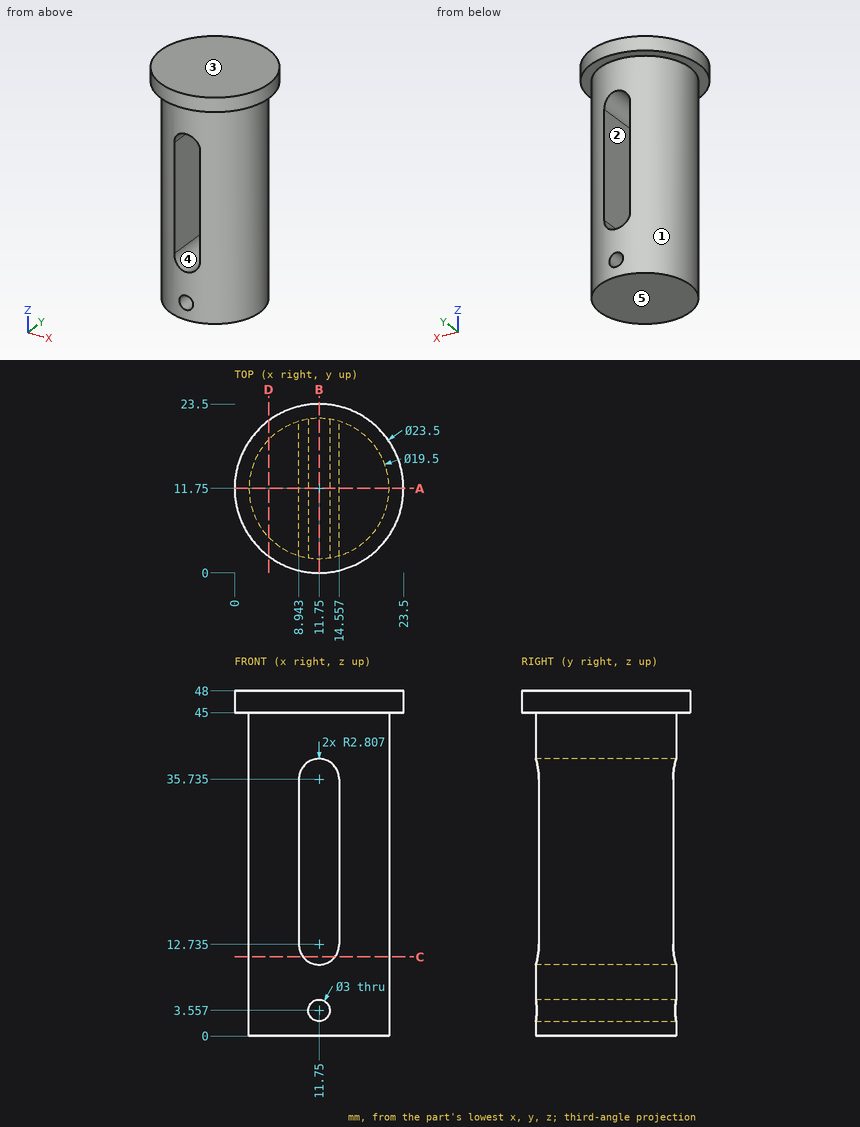
Part print with two shaded views. Sizes in mm from the minimum x, y, z corner. A direction names the side the tool comes from. Coordinates: 2 decimals unless noted, no trailing zeros. Write each loop counter-clockwise with the first axis right and the second up, starting at its lowest first coordinate (ties: lowest second). Pieces come first, ordered by that corner, then holes. Notation, with made-up numbers: (86, 30.25) - (107, 30.25) arc R12 cw to (107, 45.25) - close; hole circle Ø4 at (88, -24). An arc over 180 degrees is marked (long way). One line per item, written item: value. Start each with the question number.
1. Mould opens along Z. For the marked faces 3, 4 and 5 say: released by +Z, released by -Z, zero draft, split by the parting line, or undercut.
2. Slice it at D-D (x = 4.75). Write the cut outline in (y, z).
3. Slice it at C-C (z = 11). Write the cut outline in (x, y).
4. Flat gauge pins, fed straight in: pin 1 (5.5 mm diameter, centred on y = 16.5, z = 29, fed in from +X); pin 2 (3 mm diameter, centred on y = 10, z = 5, fed in from -X); pin 3 (5 mm diameter, centred on x = 5.5, z = 37.5, fed in from +Y). Where does each tip first touch, or does it go through?
5. Tool access for the marked faces 1 and 2: list every direction of +Z, -Z, +X, -X, +Y, -Y with a clear straight run to the whole face (end or side of a thin tool).
6. Slice it at A-A (y = 11.75). Count the separate pieces of the cut face and the enclosed holes in it, plus the area to 3 significant figures.
7. Slice it at B-B (x = 11.75). Write the cut outline in (y, z).
8. Probe line 1 (Z direction, x = 11.75, y = 12); line 2 (Z direction, x = 11, y = 11) (1 decimal); line 3 (X direction, y = 7.75, z = 13). List the from-to ranges inside material, lowest first. Write a range as from..to.
Answers below:
1. face 3: released by +Z
1. face 4: undercut
1. face 5: released by -Z
2. outline: (2.31, 45) - (4.96, 45) - (4.96, 0) - (18.54, 0) - (18.54, 45) - (21.19, 45) - (21.19, 48) - (2.31, 48) - close
3. outline: (9.54, 2.25) - (9.54, 21.25) arc R9.75 ccw to start; (13.96, 2.25) arc R9.75 ccw to (13.96, 21.25) - close
4. pin 1: stops at x = 21.29
4. pin 2: stops at x = 2
4. pin 3: stops at y = 20.75
5. face 1: -Z
5. face 2: +Y, -Y
6. separate pieces: 1
6. enclosed holes: 2
6. area: 787 mm^2
7. outline: (0, 45) - (2, 45) - (2, 38.54) - (21.5, 38.54) - (21.5, 45) - (23.5, 45) - (23.5, 48) - (0, 48) - close; (2, 0) - (21.5, 0) - (21.5, 2.06) - (2, 2.06) - close; (2, 5.06) - (21.5, 5.06) - (21.5, 9.93) - (2, 9.93) - close
8. line 1: z = 0..2.06, 5.06..9.93, 38.54..48
8. line 2: z = 0..2.3, 4.9..10, 38.4..48
8. line 3: x = 2.86..8.94, 14.56..20.64
